from build123d import *

# Parameters (mm, degrees)
F0_W      = 80
F0_H      = 70
F1_DEPTH  = 45
F2_R      = 13
F3_DEPTH  = 45.001
F4_R      = 16
F4_R_2    = 13
F5_DEPTH  = 15
F7_R      = 16.85
F8_DEPTH  = 1.3
F10_D     = 8.8
F10_DEPTH = 36
F10_TIP   = 2.6437867237


with BuildPart() as f1:
    # F0 (on Front) → F1 (new body)
    with BuildSketch(Plane.XZ):
        with Locations((40, 35)):
            Rectangle(F0_W, F0_H)
    extrude(amount=F1_DEPTH)

    # F2 (on face) → F3 (cut, through all)
    with BuildSketch(Plane.XZ.offset(45)):
        with Locations((40, 40)):
            Circle(F2_R)
    extrude(amount=-F3_DEPTH, mode=Mode.SUBTRACT)

    # F4 (on face) → F5 (cut)
    with BuildSketch(Plane.XZ.offset(45)):
        with Locations((40, 40)):
            Circle(F4_R)
        with Locations((40, 40)):
            Circle(F4_R_2, mode=Mode.SUBTRACT)
    extrude(amount=-F5_DEPTH, mode=Mode.SUBTRACT)

    # F7 (on offset) → F8 (cut)
    with BuildSketch(Plane.XZ.offset(39)):
        with Locations((40, 40)):
            Circle(F7_R)
    extrude(amount=F8_DEPTH, mode=Mode.SUBTRACT)

    # F10
    with Locations(Plane(origin=(0, 0, 0), x_dir=(1, 0, 0), z_dir=(0, 0, -1))):
        with Locations((15, 22.5), (65, 22.5)):
            Hole(F10_D / 2, depth=F10_DEPTH)
            with Locations((0, 0, -(F10_DEPTH + F10_TIP / 2))):  # 118° drill point
                Cone(0, F10_D / 2, F10_TIP, mode=Mode.SUBTRACT)


solid = f1.part
Design review of the part built by this model. Coordinates are the model's own, in mm. A direction names the side the tool comes from. Coordinates: 2 decimals unless noted, no trailing zeros. Write each loop counter-clockwise with the first axis right and the second up, starting at its lowest first coordinate (ties: lowest second). Pieces come first, ordered by that corner, then holes. Notation, with made-up numbers: (-3, 67.25) - (4, 67.25) arc R20 cw to (4, 98.25) - close; hole circle Ø1 at (51.25, 19). An arc over 180 degrees is marked (long way). One line per item, written item: value.
1) To check wall thickness, follow probe 1 along X at (y, z) = (-22.5, 21.5); probe 2 along Z at (x, y) = (40, -6); probe 3 along X at (y, z) = (-25.5, 10). State the ranges of each line that lie inside material, in increasing order.
Answer sheet:
probe 1: x = 0 to 10.6, 19.4 to 60.6, 69.4 to 80
probe 2: z = 0 to 27, 53 to 70
probe 3: x = 0 to 11.78, 18.22 to 61.78, 68.22 to 80
2) Insertion check: pin 1 (7 mm diameter, centred on x = 65, y = -22.5, fed in from -Z); pin 2 (1.5 mm diameter, centred on x = 15.5, y = -22.5, fed in from -Z). Each pin has a flat end and moves straight along its axis. Give the tip position at first contact, or say it passes through.
Answer sheet:
pin 1: stops at z = 36.54
pin 2: stops at z = 37.89
3) Add section B-B (z = 35). State the section outline as (x, y) points.
Answer sheet:
outline: (0, -45) - (24.8, -45) - (24.8, -40.3) - (23.91, -40.3) - (23.91, -39) - (24.8, -39) - (24.8, -30) - (28, -30) - (28, 0) - (0, 0) - close; (52, -30) - (55.2, -30) - (55.2, -39) - (56.09, -39) - (56.09, -40.3) - (55.2, -40.3) - (55.2, -45) - (80, -45) - (80, 0) - (52, 0) - close; hole circle Ø8.8 at (15, -22.5); hole circle Ø8.8 at (65, -22.5)
4) Mouldability with a two-part tool opening along Z and no side actions: class faces 1 (the face through (69.396, -22.693, 18.252)), 2 (the face through (39, -22, 70)), 3 (the face through (38.7, -30, 53.1)) as +Z half, -Z half, draft (parallel to the pull), parting line (faces both ways), or undercut.
Answer sheet:
face 1: draft
face 2: +Z half
face 3: undercut
5) Add section C-C (y = -36.5). State the section outline as (x, z) points.
Answer sheet:
outline: (0, 0) - (80, 0) - (80, 70) - (0, 70) - close; hole circle Ø32 at (40, 40)
6) Add section A-A (x = 40). State the section outline as (y, z) points, plus the area to 3 significant figures.
Answer sheet:
outline: (-45, 0) - (0, 0) - (0, 27) - (-30, 27) - (-30, 24) - (-39, 24) - (-39, 23.15) - (-40.3, 23.15) - (-40.3, 24) - (-45, 24) - close; (-45, 56) - (-40.3, 56) - (-40.3, 56.85) - (-39, 56.85) - (-39, 56) - (-30, 56) - (-30, 53) - (0, 53) - (0, 70) - (-45, 70) - close
area: 1,890 mm2
7) Add section D-D (z = 9). State the section outline as (x, y) points.
Answer sheet:
outline: (0, -45) - (80, -45) - (80, 0) - (0, 0) - close; hole circle Ø8.8 at (15, -22.5); hole circle Ø8.8 at (65, -22.5)
8) For faces 4 (the face through (24.015, -34.563, 40.703)), 5 (the face through (10.803, -23.822, 18.252)), 6 (the face through (49.058, -39.641, 54.208)), list the 3-axis set-ups (+Z, -Z, +X, -X, +Y, -Y) from which the entire face can be reached by the end or side of a thin tool; tool diameter is ignored.
Answer sheet:
face 4: -Y
face 5: -Z
face 6: none
